Answer from the drawing. Dimensions are ordinates in mm from the lowest x, y and z of the part. A direction names the side the tool comes from. Give positions to 0.01 mm unless a question says otherwise; leave off trailing zeros. Write each loop counter-clockwise with the first axis right and the second up, starting at its lowest first coordinate (ties: lowest second). Pieces come first, ordered by that corner, then holes. Notation, with made-up numbers: (48.25, -10) - (101.25, -10) arc R25 ccw to (101.25, 2) - close; hole circle Ø5 at (80.5, -15.5). An arc over 180 degrees is marked (long way). Answer as a JSON object with one key per item and string values. Group by question number.
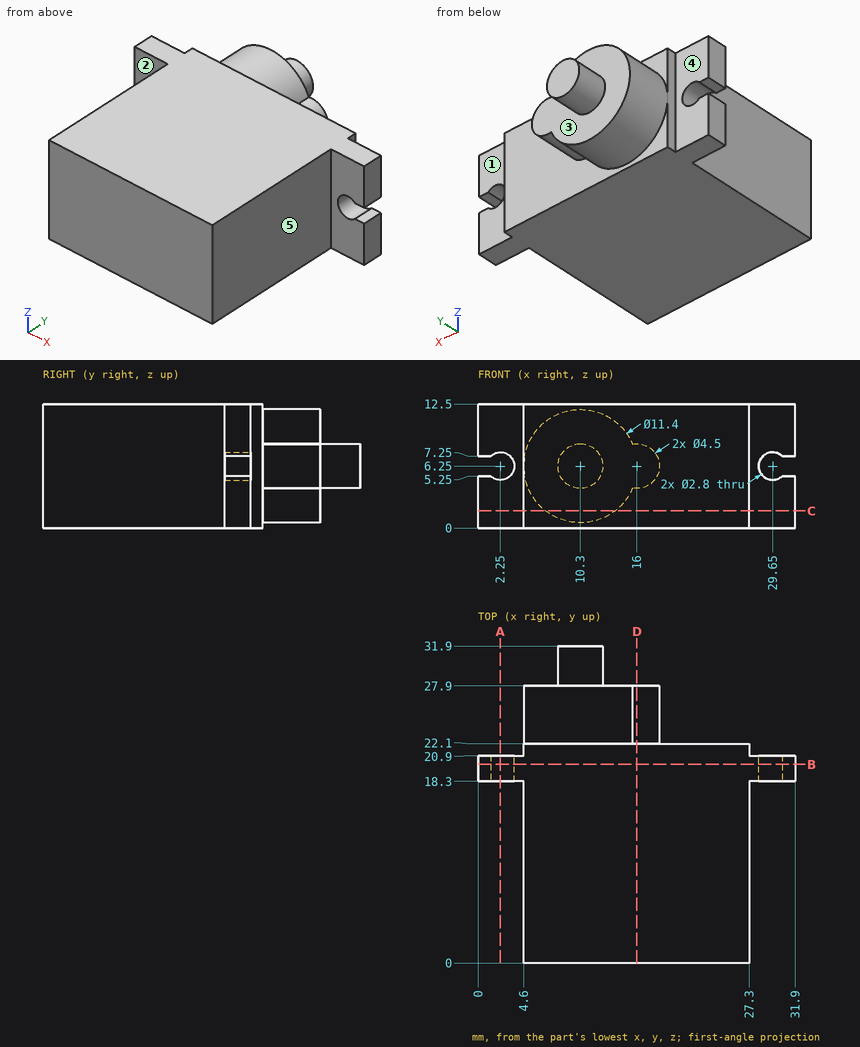
1) Find section C-C, the plane z = 1.75. Write down the section's boundary in (x, y), and give its area (3 significant figures).
2) Find the intervals of material crossed by line 1 (Z direction, x = 29.65, y = 18.95); line 2 (X direction, y = 3.5, z = 11); line 3 (X direction, y = 20.2, z = 6.25), in increasing order. Write a range as [from, to].
3) Find section A-A, the plane x = 2.25. Write down the section's boundary in (y, z), and give its area (3 significant figures).
4) Flat-ended cylindrical pins translate along their axes: pin 1 Ø5 at (x, z) = (30.5, 4.5) entering from -Y; pin 2 Ø5 at (x, y) = (18, 26) entering from -Z; pin 3 Ø3.5 at (x, z) = (1.5, 3) entering from +Y; pin 4 Ø2 at (x, z) = (29.65, 6.25) entering from +Y. Find the tip coordinate at first contact, or state that the pin passes through.
5) Find section B-B, the plane y = 20. Write down the section's boundary in (x, z), and give its area (3 significant figures).
6) Which of the six approach directions +Z, -Z, +X, -X, +Y, -Y give full straight-line access (tool end or side, diameter ignored) to the marked faces 1, 2, 3, 4 and 5?
7) Find section D-D, the plane x = 16. Write down the section's boundary in (y, z), and give its area (3 significant figures).
Values follow:
{
 "1": {"outline": "(0, 18.3) - (4.6, 18.3) - (4.6, 0) - (27.3, 0) - (27.3, 18.3) - (31.9, 18.3) - (31.9, 20.9) - (27.3, 20.9) - (27.3, 22.1) - (13.8, 22.1) - (13.8, 27.9) - (6.8, 27.9) - (6.8, 22.1) - (4.6, 22.1) - (4.6, 20.9) - (0, 20.9) - close", "area": "566 mm2"},
 "2": {"line 1": "z = [0, 4.85], [7.65, 12.5]", "line 2": "x = [4.6, 27.3]", "line 3": "x = [3.65, 28.25]"},
 "3": {"outline": "(18.3, 0) - (20.9, 0) - (20.9, 4.85) - (18.3, 4.85) - close; (18.3, 7.65) - (20.9, 7.65) - (20.9, 12.5) - (18.3, 12.5) - close", "area": "25.2 mm2"},
 "4": {"pin 1": "stops at y = 18.3", "pin 2": "stops at z = 3.92", "pin 3": "stops at y = 20.9", "pin 4": "passes through"},
 "5": {"outline": "(0, 0) - (31.9, 0) - (31.9, 5.25) - (30.63, 5.25) arc R1.4 cw (long way) to (30.63, 7.25) - (31.9, 7.25) - (31.9, 12.5) - (0, 12.5) - (0, 7.25) - (1.27, 7.25) arc R1.4 cw (long way) to (1.27, 5.25) - (0, 5.25) - close", "area": "383 mm2"},
 "6": {"face 1": "+Z, -Z, +X, +Y", "face 2": "+Z, -Z, -X, -Y", "face 3": "+Y", "face 4": "+Z, -Z, -X, +Y", "face 5": "+Z, -Z, +X, -Y"},
 "7": {"outline": "(0, 0) - (22.1, 0) - (22.1, 4) - (27.9, 4) - (27.9, 8.5) - (22.1, 8.5) - (22.1, 12.5) - (0, 12.5) - close", "area": "302 mm2"}
}
